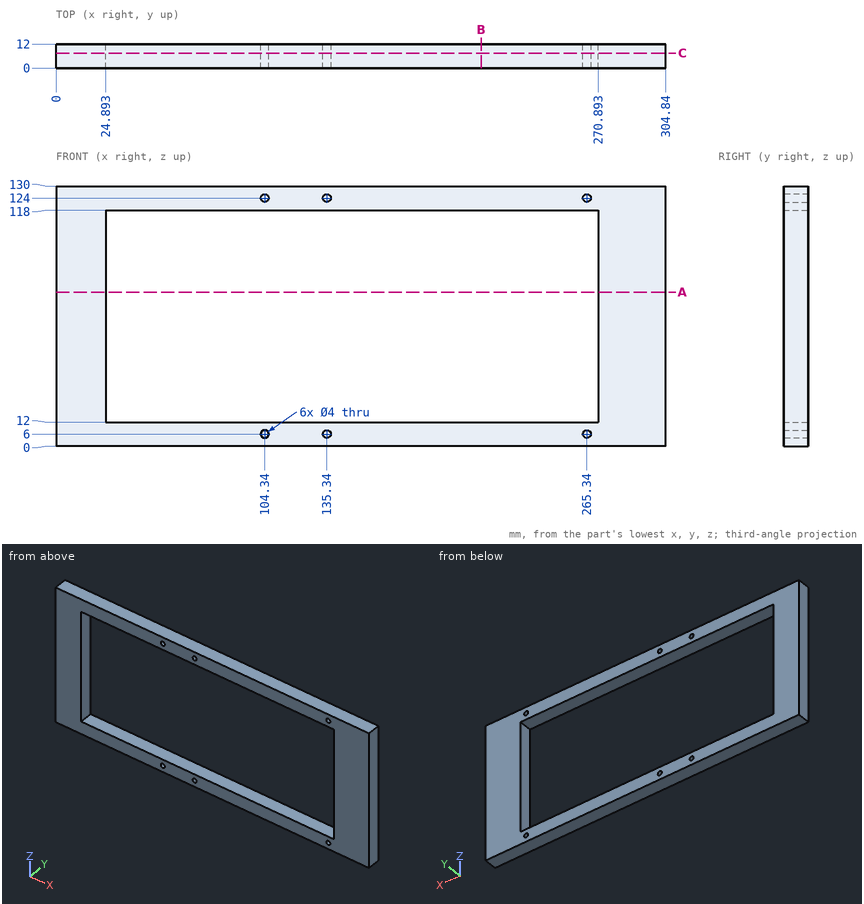
Answer from the drawing. Dimensions are ordinates in mm from the lowest x, y and z of the part. Give positions to 0.01 mm unless a question says otherwise; leave off trailing zeros. Order: outer loops, then holes, each group sorted by start corner. A loop starts at its lowest first (then second) coordinate and runs counter-clockwise, first axis right, second up. Notation, with made-up numbers: (-22, -26.75) - (9, -26.75) arc R17 cw to (9, -21.75) - close; hole circle Ø6 at (34.5, 45). An arc over 180 degrees is marked (long way). Use one line per item in the form item = value.
1) Each of these flat-tipped pins is pushed along its axis until it touches: pin 1 (5 mm diameter, centred on x = 135.34, z = 6, fed in from -Y); pin 2 (3 mm diameter, centred on x = 265.34, z = 6, fed in from +Y). Where does it stop, or does it pass through?
Verdict:
pin_1 = 0
pin_2 = through
2) Find section C-C on y = 7.5. Determine the outline of the cut face in (x, z), and give its area (3 significant figures).
Verdict:
outline = (0, 0) - (304.84, 0) - (304.84, 130) - (0, 130) - close; hole (24.89, 12) - (270.89, 12) - (270.89, 118) - (24.89, 118) - close; hole circle Ø4 at (104.34, 6); hole circle Ø4 at (104.34, 124); hole circle Ø4 at (135.34, 6); hole circle Ø4 at (135.34, 124); hole circle Ø4 at (265.34, 6); hole circle Ø4 at (265.34, 124)
area = 13,500 mm^2
3) Find section A-A on z = 77. Determine the outline of the cut face in (x, y).
Verdict:
outline = (0, 0) - (24.89, 0) - (24.89, 12) - (0, 12) - close; (270.89, 0) - (304.84, 0) - (304.84, 12) - (270.89, 12) - close
4) Find section B-B on x = 212.5. Determine the outline of the cut face in (y, z), and give its area (3 significant figures).
Verdict:
outline = (0, 0) - (12, 0) - (12, 12) - (0, 12) - close; (0, 118) - (12, 118) - (12, 130) - (0, 130) - close
area = 288 mm^2
5) Consider probe 1 along X at (y, z) = (5.5, 6); probe 2 along Z at (x, y) = (135.5, 7.25); probe 3 along X at (y, z) = (4.5, 108). Determine where each line is inside the solid, lowest interval first. Write a range as [from, to].
Verdict:
probe_1 = [0, 102.34], [106.34, 133.34], [137.34, 263.34], [267.34, 304.84]
probe_2 = [0, 4.01], [7.99, 12], [118, 122.01], [125.99, 130]
probe_3 = [0, 24.89], [270.89, 304.84]
